For this review, take the finished solid that the model builds, in its own axes (mm). A direction names the side the tool comes from. Round coordinates to 2 decimals unless told otherwise and drop trailing zeros. Order: outer loops, then holes, each group sorted by start corner. A loop starts at its lowest first (then second) coordinate and runs counter-clockwise, first axis right, second up. Notation, with made-up numbers: (-0.75, -21) - (54.25, -21) arc R26 ccw to (54.25, -5) - close; hole circle Ø7 at (-6.5, 25.25). An arc over 180 degrees is marked (long way). One line per question, with ' | ' between items.
```python
from build123d import *

# Parameters (mm, degrees)
F0_W     = 276.225
F0_H     = 19.05
F0_W_2   = 19.05
F0_H_2   = 419.1
F1_DEPTH = 152.4


with BuildPart() as f1:
    # F0 (on Top) → F1 (new body)
    with BuildSketch(Plane.XY):
        Polygon((-473.202007, 368.503202), (-492.252007, 368.503202), (-492.252007, -50.596798), (-473.202007, -50.596798), (-473.202007, 158.953202), (-473.202007, 178.003202), align=None)
        with Locations((-335.089507, 168.478202)):
            Rectangle(F0_W, F0_H)
        Polygon((117.347993, 387.553202), (-492.252007, 387.553202), (-492.252007, 368.503202), (-473.202007, 368.503202), (-196.977007, 368.503202), (-177.927007, 368.503202), (98.297993, 368.503202), (117.347993, 368.503202), align=None)
        Polygon((-177.927007, 368.503202), (-196.977007, 368.503202), (-196.977007, 178.003202), (-196.977007, 158.953202), (-196.977007, -50.596798), (-177.927007, -50.596798), align=None)
        with Locations((107.822993, 158.953202)):
            Rectangle(F0_W_2, F0_H_2)
        Polygon((-473.202007, -50.596798), (-492.252007, -50.596798), (-492.252007, -69.646798), (117.347993, -69.646798), (117.347993, -50.596798), (98.297993, -50.596798), (-177.927007, -50.596798), (-196.977007, -50.596798), align=None)
    extrude(amount=F1_DEPTH)


solid = f1.part
```
(1) We need section A-A on x = 77.5. State the section outline as (y, z) points, plus the area to 3 significant figures.
Output values:
outline: (-69.65, 0) - (-50.6, 0) - (-50.6, 152.4) - (-69.65, 152.4) - close; (368.5, 0) - (387.55, 0) - (387.55, 152.4) - (368.5, 152.4) - close | area: 5,810 mm^2
(2) We need section B-B on y = 228.5. State the section outline as (x, z) points.
Output values:
outline: (-492.25, 0) - (-473.2, 0) - (-473.2, 152.4) - (-492.25, 152.4) - close; (-196.98, 0) - (-177.93, 0) - (-177.93, 152.4) - (-196.98, 152.4) - close; (98.3, 0) - (117.35, 0) - (117.35, 152.4) - (98.3, 152.4) - close
(3) We need section C-C on z = 46. State the section outline as (x, y) points.
Output values:
outline: (-492.25, -69.65) - (117.35, -69.65) - (117.35, 387.55) - (-492.25, 387.55) - close; hole (-473.2, -50.6) - (-196.98, -50.6) - (-196.98, 158.95) - (-473.2, 158.95) - close; hole (-473.2, 178) - (-196.98, 178) - (-196.98, 368.5) - (-473.2, 368.5) - close; hole (-177.93, -50.6) - (98.3, -50.6) - (98.3, 368.5) - (-177.93, 368.5) - close
(4) For probe 1 along X at (y, z) = (298.5, 107); probe 2 along Y at (x, z) = (-235, 121.5); probe 3 along X at (y, z) = (165, 84), list the stretches that pass through material, from the lowest coordinate up. Write a range as [from, to].
Output values:
probe 1: [-492.25, -473.2], [-196.98, -177.93], [98.3, 117.35] | probe 2: [-69.65, -50.6], [158.95, 178], [368.5, 387.55] | probe 3: [-492.25, -177.93], [98.3, 117.35]
(5) For faces 4 (the flat face through (-333, -50.597, 75)), 5 (the flat face through (-211, 177, 152.4)), list the 3-axis set-ups (+Z, -Z, +X, -X, +Y, -Y) from which the entire face can be reached by the end or side of a thin tool; tool diameter is ignored.
Output values:
face 4: +Z, -Z | face 5: +Z, +X, -X, +Y, -Y
(6) Mouldability with a two-part tool opening along Y and no side actions: class faces 1 (the flat face through (-183, 387.553, 75)), 2 (the flat face through (117.348, 156, 75)), 3 (the flat face through (-38, -50.597, 75)) as released by +Y, released by -Y, zero draft, split by the parting line, or undercut.
Output values:
face 1: released by +Y | face 2: zero draft | face 3: undercut
